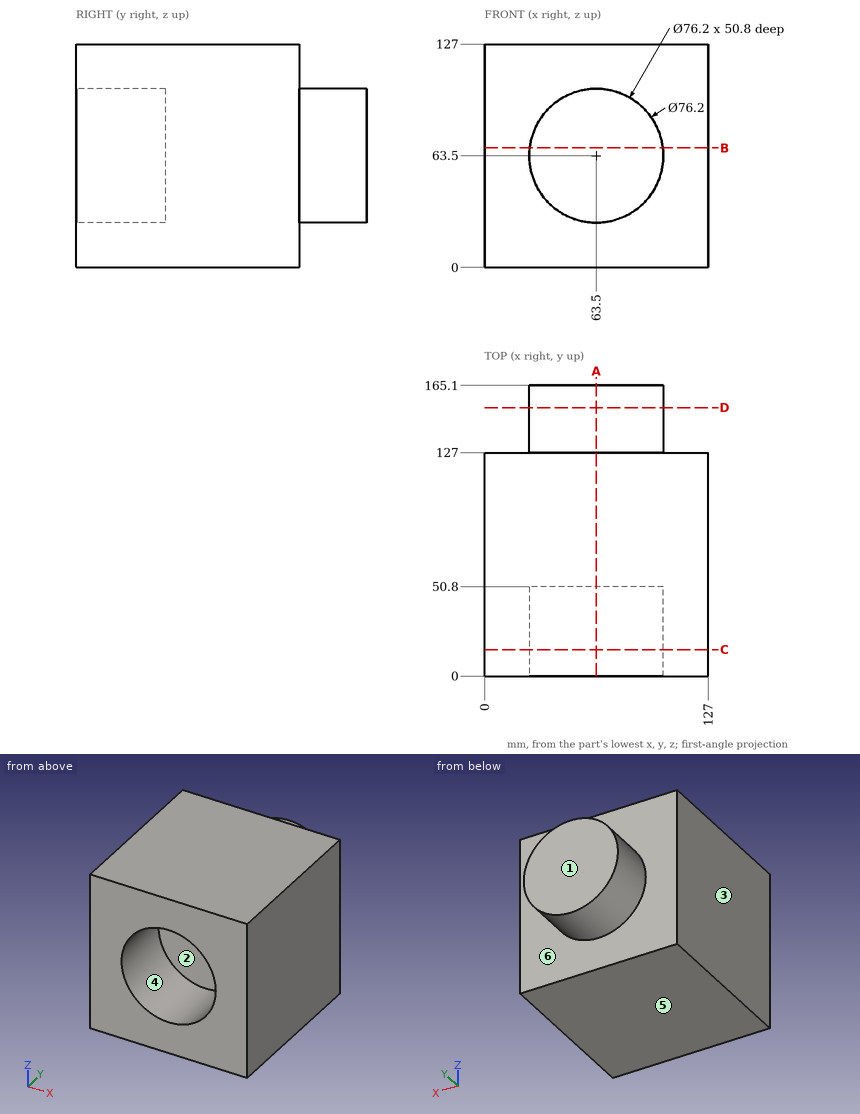
Verification items for this drawing (mm, ordinates from the low corner). A direction names the side the tool comes from. Give positions to 0.01 mm unless a question says otherwise; leave off trailing zeros. Write each loop counter-clockwise with the first axis right and the second up, starting at its lowest first coordinate (ties: lowest second). Pieces come first, ordered by that corner, then holes. Notation, with made-up numbers: (71.5, -4.75) -> (95.5, -4.75) arc R27 ccw to (95.5, 12.25) -> close; hole circle Ø5 at (76.5, 64.25). An arc over 180 degrees is marked (long way). Use CSV: the item, a comma, the result in double quotes. Start each with the question number.
Q1. Cross-section at D-D on y = 152.5. Enter the section's corners in (x, z).
Q2. Scan lines: line 1 along Z through (x, y) = (63.5, 35); line 2 along Y through (x, z) = (76, 98); line 3 along Y through (x, z) = (118, 99). Record each from-to range of solid material in increasing order.
Q3. Depth check by flat-ended pin: P1, Ø2, axis at x = 102, z = 28, coming from the -Y side; P2, Ø8, axis at x = 18.5, z = 87.5, coming from the +Y side; P3, Ø8, axis at x = 79.5, z = 78, coming from the -Y side. Enter the tip coordinate at first touch or a pass-through.
Q4. Release check for a two-part mould opening along X. For the marked faces 1, 2 and 3 record: +X half, -X half, draft (parallel to the pull), parting line (faces both ways), or undercut.
Q5. Cross-section at B-B on z = 68. Enter the section's corners in (x, y), and give its area (3 significant figures).
Q6. Cross-section at C-C on y = 15. Enter the section's corners in (x, z).
Q7. Cross-section at A-A on x = 63.5. Enter the section's corners in (y, z).
Q8. Tool access check on the marked faces 4, 5 and 6. Record the directions out of +Z, -Z, +X, -X, +Y, -Y that give a thin tool (end or side, any length) a straight path to the whole face; none if there is none.
Working result:
1,outline,"circle Ø76.2 at (63.5, 63.5)"
2,line 1,"z = 0 to 25.4, 101.6 to 127"
2,line 2,"y = 50.8 to 165.1"
2,line 3,"y = 0 to 127"
3,P1,"stops at y = 0"
3,P2,"stops at y = 127"
3,P3,"stops at y = 50.8"
4,face 1,"draft"
4,face 2,"undercut"
4,face 3,"-X half"
5,outline,"(0, 0) -> (25.67, 0) -> (25.67, 50.8) -> (101.33, 50.8) -> (101.33, 0) -> (127, 0) -> (127, 127) -> (101.33, 127) -> (101.33, 165.1) -> (25.67, 165.1) -> (25.67, 127) -> (0, 127) -> close"
5,area,"15,200 mm^2"
6,outline,"(0, 0) -> (127, 0) -> (127, 127) -> (0, 127) -> close; hole circle Ø76.2 at (63.5, 63.5)"
7,outline,"(0, 0) -> (127, 0) -> (127, 25.4) -> (165.1, 25.4) -> (165.1, 101.6) -> (127, 101.6) -> (127, 127) -> (0, 127) -> (0, 101.6) -> (50.8, 101.6) -> (50.8, 25.4) -> (0, 25.4) -> close"
8,face 4,"-Y"
8,face 5,"-Z, +X, -X, +Y, -Y"
8,face 6,"+Y"
